Source: CAD feature listing. Evaluate the final solid. Frame: model axes, mm. Round coordinates to 2 decimals unless told otherwise and drop trailing zeros. Answer in a Markdown table with one row per item.
Autodesk Inventor part; units mm, degrees
ref_plane "YZ Plane" through (0, 0, 0) normal (1, 0, 0) x (0, 1, 0)
ref_plane "XZ Plane" through (0, 0, 0) normal (0, 1, 0) x (-1, 0, 0)
ref_plane "XY Plane" through (0, 0, 0) normal (0, 0, 1) x (1, 0, 0)
sketch "Sketch1" plane through (0, 0, 0) normal (0, 1, 0) x (-1, 0, 0)
  line L0 (0, 0) -> (10.5, 0)
  line L1 (10.5, 0) -> (10.5, -10.5)
  line L2 (10.5, -10.5) -> (0, -10.5)
  line L3 (0, -10.5) -> (0, 0)
  dimension "d0" = 10.5
  dimension "d1" = 10.5
extrude "Extrusion1" add sketch "Sketch1" along normal blind 20
sketch "Sketch2" plane through (0, 20, 0) normal (0, 1, 0) x (1, 0, 0)
  line L0 (0, 0) -> (-2, 0)
  line L1 (-2, 0) -> (-2, 2.625)
  line L2 (-2, 2.625) -> (0, 2.625)
  line L3 (0, 2.625) -> (0, 0)
  line L4 (-2, 2.625) -> (-6, 2.625)
  line L5 (-6, 2.625) -> (-6, 7.875)
  line L6 (-6, 7.875) -> (-2, 7.875)
  line L7 (-2, 7.875) -> (-2, 2.625)
  line L8 (-6, 2.625) -> (-8, 2.625) construction
  line L9 (-8, 2.625) -> (-8, 1.625) construction
  line L10 (-8, 1.625) -> (-6, 1.625) construction
  line L11 (-6, 1.625) -> (-6, 2.625)
  line L12 (-6, 1.625) -> (-8, 1.625)
  line L13 (-8, 1.625) -> (-8, 8.875) construction
  line L14 (-8, 8.875) -> (-6, 8.875)
  line L15 (-6, 8.875) -> (-6, 1.625)
  line L16 (-8, 5.25) -> (-6, 1.625)
  line L17 (-8, 5.25) -> (-6, 8.875)
  dimension "d4" = 2
  dimension "d5" = 2.625
  dimension "d6" = 4
  dimension "d7" = 5.25
  dimension "d8" = 2
  dimension "d9" = 1
  dimension "d10" = 2
  dimension "d11" = 7.25
extrude "Extrusion2" cut sketch "Sketch2" against normal blind 0.2 contours L4 L5 L6 L7 | L11 L16 L17 L15 L5
properties part number "Air_heater_button"
Q1. Contact query for a flat-ended pin moving along its axis: pin 1 Ø1 at (x, y) = (-3.5, 17) entering from +Z. Output: stop coordinate, or through.
Solutions:
| item | result |
|---|---|
| pin 1 | stops at z = 0 |
Q2. Pull-direction query (Z, two-part tool) for faces 1 (the flat face through (-5, 10, -10.5)), 2 (the flat face through (-5, 10, 0)), 3 (the flat face through (-4, 19.8, -5)), 4 (the flat face through (0, 10, -5)); classes: pulls with the +Z half, pulls with the -Z half, needs draft (parallel to the pull), parting line crosses it, or undercut.
Solutions:
| item | result |
|---|---|
| face 1 | pulls with the -Z half |
| face 2 | pulls with the +Z half |
| face 3 | undercut |
| face 4 | needs draft |
Q3. Material intervals for probe 1 along Y at (x, z) = (-5.5, -4), sorted ascending.
Solutions:
| item | result |
|---|---|
| probe 1 | y = 0 to 19.8 |
